CAD build for the part. Positions are in the model's coordinates, mm. A direction names the side the tool comes from. Coordinates: 2 decimals unless noted, no trailing zeros. Order: outer loops, then holes, each group sorted by start corner. A loop starts at its lowest first (then second) coordinate and runs counter-clockwise, first axis right, second up. Notation, with made-up numbers: M -10.75,65 L 9.25,65 A24 cw 9.25,82 Z; hole C 73.25,80 d10. An arc over 180 degrees is marked long. Write item = value, one per line.
Autodesk Inventor part; units mm, degrees
ref_plane "Plano de trabalho4" through (29, 0, 0) normal (1, 0, 0) x (0, 1, 0)
ref_plane "XZ Plane" through (0, 0, 0) normal (0, 1, 0) x (-1, 0, 0)
ref_plane "XY Plane" through (0, 0, 0) normal (0, 0, 1) x (1, 0, 0)
sketch "Esboço1" plane through (0, 0, 0) normal (0, 0, 1) x (1, 0, 0)
  circle A0 centre (0, 0) radius 15.5
  dimension "d0" = 31
extrude "Extrusão1" add sketch "Esboço1" along normal blind 2
sketch "Esboço2" plane through (0, 0, 2) normal (0, 0, 1) x (1, 0, 0)
  circle A0 centre (0, 0) radius 15.5
  circle A1 centre (0, 0) radius 13.5
  dimension "d3" = 2
extrude "Extrusão2" add sketch "Esboço2" along normal blind 58
ref_plane "Plano de trabalho4" through (29, 0, 0) normal (1, 0, 0) x (0, 1, 0)
sketch "Esboço5" plane through (29, 0, 0) normal (1, 0, 0) x (0, 1, 0)
  line L0 (-7.75, 27) -> (7.75, 27)
  line L1 (7.75, 27) -> (7.75, 6.5)
  line L2 (7.75, 6.5) -> (-7.75, 6.5)
  line L3 (-7.75, 6.5) -> (-7.75, 27)
  line L4 (-7.75, 27) -> (7.75, 6.5) construction
  line L5 (7.75, 27) -> (-7.75, 6.5) construction
  line L6 (15.5, 0) -> (-15.5, 0)
  point P0 (0, 0)
  point P1 (0, 16.75)
  dimension "d15" = 20.5
  dimension "d16" = 15.5
  dimension "d17" = 0
  dimension "d18" = 6.5
extrude "Extrusão4" cut sketch "Esboço5" against normal through all
sketch "Esboço7" plane through (0, 0, 60) normal (0, 0, 1) x (1, 0, 0)
  circle A0 centre (0, 0) radius 16.5
  circle A1 centre (0, 0) radius 13.5
  dimension "d28" = 33
extrude "Extrusão6" add sketch "Esboço7" along normal blind 2
fillet "Arredondamento2" radius 2 1 edges at (-13.5, 0, 62)
fillet "Arredondamento3" radius 2 1 edges at (-15.5, 0, 60)
sketch "Sketch8" plane through (0, 0, 0) normal (1, 0, 0) x (0, 1, 0)
  line L0 (-9.75, 21.75) -> (9.75, 21.75)
  line L1 (9.75, 21.75) -> (9.75, 23.25)
  line L2 (9.75, 23.25) -> (-9.75, 23.25)
  line L3 (-9.75, 23.25) -> (-9.75, 21.75)
  line L4 (-7.75, 27) -> (7.75, 27)
  line L5 (7.75, 27) -> (7.75, 6.5)
  line L6 (-7.75, 6.5) -> (-7.75, 27)
  point P0 (0, 0)
  dimension "d37" = 3.75
  dimension "d38" = 1.5
  dimension "d39" = 2
  dimension "d40" = 2
extrude "Extrusion7" cut sketch "Sketch8" along normal mid plane 50 contours L3 L2 L6 L0 | L6 L2 L5 L0 | L5 L2 L1 L0
sketch "Sketch11" plane through (0, 0, 0) normal (0, 0, -1) x (-1, 0, 0)
  line L0 (-18.5, -10) -> (-15.5, -10)
  line L1 (-15.5, -10) -> (-15.5, 10)
  line L2 (-15.5, 10) -> (-18.5, 10)
  line L3 (-18.5, 10) -> (-18.5, -10)
  circle A0 centre (0, 0) radius 16.5
  point P0 (-16.5, 0)
  point P1 (-15.5, 5.6569)
  point P2 (-15.5, -5.6569)
  dimension "d48" = 3
  dimension "d49" = 2
  dimension "d50" = 20
  dimension "d51" = 10
extrude "Extrusion9" add sketch "Sketch11" against normal blind 5
fillet "Fillet4" radius 1 2 edges at (15.5, 5.6569, 2.5) (15.5, -5.6569, 2.5)
properties part number "peca1v2"
(1) Slice it at D-D, the plane y = -6. State how many separate pieces and enclosed holes the cut face has, then the cut area to 3 significant figures.
Evaluation:
separate_pieces = 3
enclosed_holes = 0
area = 333 mm²
(2) Slice it at A-A, the plane y = 0. Write the cut outline in (x, z).
Evaluation:
outline = M -16.5,0 L 18.5,0 L 18.5,5 L 15.5,5 L 15.5,6.5 L 13.5,6.5 L 13.5,5 L -13.5,5 L -13.5,6.5 L -15.5,6.5 L -15.5,5 L -16.5,5 Z; M -16.5,60 A2 cw -15.5,58.27 L -15.5,27 L -13.5,27 L -13.5,60 A2 ccw -15.5,62 L -16.5,62 Z; M 13.5,27 L 15.5,27 L 15.5,58.27 A2 cw 16.5,60 L 16.5,62 L 15.5,62 A2 ccw 13.5,60 Z
(3) Pin check, flat tips, straight feed: pin 1 Ø3.5 at (x, y) = (13, 2) entering from +Z; pin 2 Ø6 at (x, y) = (12, 2) entering from -Z; pin 3 Ø2.5 at (x, z) = (12.5, 14.5) entering from +Y; pin 4 Ø10 at (x, y) = (-4, 2.5) entering from +Z. Stop position of each tip, or through.
Evaluation:
pin_1 = 61.91
pin_2 = 0
pin_3 = 10.66
pin_4 = 5
(4) Slice it at B-B, the plane x = 0. Write the cut outline in (y, z), then the cut area to 3 significant figures.
Evaluation:
outline = M -16.5,0 L 16.5,0 L 16.5,5 L 15.5,5 L 15.5,58.27 A2 cw 16.5,60 L 16.5,62 L 15.5,62 A2 ccw 13.5,60 L 13.5,5 L -13.5,5 L -13.5,60 A2 ccw -15.5,62 L -16.5,62 L -16.5,60 A2 cw -15.5,58.27 L -15.5,5 L -16.5,5 Z
area = 396 mm²
(5) Slice it at C-C, the plane z = 47. Write the cut outline in (x, y).
Evaluation:
outline = C 0,0 d31; hole C 0,0 d27
(6) Wall check: line 1 (X direction, y = 0, z = 40); line 2 (Z direction, x = 15, y = 3). Give the ranges that are in metal, low to high. Write a range as from..to.
Evaluation:
line_1 = -15.5..-13.5, 13.5..15.5
line_2 = 0..6.5, 27..61.99
(7) Tool access for faces 1 (the face through (14, 0, 27)), 2 (the face through (0, 0, 5)), 3 (the face through (17, -10, 2)), 4 (the face through (-15.485, -0.682, 31.261)), 5 (the face through (-16.49, -0.59, 2.46)): list every direction of +Z, -Z, +X, -X, +Y, -Y with a clear straight run to the whole face (end or side of a thin tool).
Evaluation:
face_1 = +X, -X
face_2 = +Z
face_3 = +Z, -Z, +X, -Y
face_4 = none
face_5 = +Z, -Z
(8) Pull direction Y, two halves, no side cores. Call faces 6 (the face through (17, 10, 2)), 7 (the face through (11, -9, 23.25)), 8 (the face through (-15, -5, 62)): +Y half, -Y half, draft (parallel to the pull), parting line (faces both ways), or undercut.
Evaluation:
face_6 = +Y half
face_7 = undercut
face_8 = draft
